Geometry: final body of the model. Coordinates: model frame, mm. Face numbers are marked on the shaded views. A direction names the side the tool comes from. Give positions to 0.01 mm unless a question says otherwise; leave off trailing zeros. Loops run counter-clockwise (first coordinate to the right, second up) from the corner with the lowest first, then second, coordinate; pieces in that order, holes last. Notation, with made-up numbers: (11, 89) -> (21, 89) arc R23 ccw to (21, 116) -> close; hole circle Ø5 at (19.25, 2.25). An arc over 180 degrees is marked (long way). Answer in a Markdown table with one row per item. Add a question column.
1) Line query: line 1 (Z direction, x = 0, y = 24.6); line 2 (Z direction, x = -2.5, y = 0.5); line 3 (X direction, y = -22.5, z = -2.5). Output: solid intervals per line, ascending. Write a range as from..to.
2) Section query B-B (y = -22.5). Return the cut outline in (x, z), plus the area to 3 significant figures.
3) First-contact query: P1, Ø10, axis at y = -2, z = -31.5, coming from the +X side; P2, Ø4, axis at y = 18.5, z = 0.5, coming from the -X side; P3, Ø2.5, axis at y = -20, z = -6, coming from the -X side; P4, Ø12, axis at y = -19.5, z = -26, coming from the -X side. Flat tips, straight axial feed; report the tip coordinate or a pass-through.
4) Section query A-A (x = 0). Give the number of separate pieces and of enclosed holes in the cut face, plus the area to 3 significant figures.
5) Section query D-D (z = -6). Return the cut outline in (x, y), plus the area to 3 significant figures.
6) Section query C-C (x = 14). Return the cut outline in (y, z), plus the area to 3 significant figures.
7) Access query for the marked faces 1, 2, 3 and 4. Directions: +Z, -Z, +X, -X, +Y, -Y. A direction counts if a zero-diameter tool reaches every point of the face in a straight line with its end or side. Return the directions, or none.
8) Draft query along Z for the marked faces 5, 6 and 7. Return one class per face: +Z half, -Z half, draft (parallel to the pull), parting line (faces both ways), or undercut.
```python
from build123d import *

# Parameters (mm, degrees)
SKETCH_1_R           = 20
EXTRUDE_1_DEPTH      = 5
SKETCH_3_W           = 18
SKETCH_3_H           = 8
EXTRUDE_2_DEPTH      = 15
EXTRUDE_3_DEPTH      = 35.22
EXTRUDE_3_DEPTH_BACK = 4.78
SKETCH_4_R           = 20
EXTRUDE_4_DEPTH      = 6
EXTRUDE_4_DEPTH_BACK = 36.43845651
SKETCH_6_R           = 15
SKETCH_10_R          = 8
CUT_EXTRUDE_1_DEPTH  = 6
EXTRUDE_START        = 6
SKETCH_14_R          = 15
EXTRUDE_6_DEPTH      = 6
CUT_EXTRUDE_START    = 6
SKETCH_11_R          = 8
CUT_EXTRUDE_4_DEPTH  = 6
SKETCH_16_R          = 4
CUT_EXTRUDE_5_DEPTH  = 50
SKETCH_23_R          = 4.01
SKETCH_23_R_2        = 3.99
EXTRUDE_7_DEPTH      = 3.22


with BuildPart() as part:
    # Sketch 1 → Extrude 1 (new body)
    with BuildSketch(Plane.XY):
        Circle(SKETCH_1_R)
    extrude(amount=EXTRUDE_1_DEPTH)

    # Sketch 3 → Extrude 2 (add)
    with BuildSketch(Plane.XY.offset(5)):
        with Locations((0, -19.652481849)):
            Rectangle(SKETCH_3_W, SKETCH_3_H)
        with Locations((0, 18.785974665)):
            Rectangle(SKETCH_3_W, SKETCH_3_H)
    extrude(amount=-EXTRUDE_2_DEPTH)

    # Sketch 4 → Extrude 3 (add, two sides: drawn at the far end of the back side and taken through both)
    with BuildSketch(Plane.XZ.offset(-14.785974665).offset(-EXTRUDE_3_DEPTH_BACK)):
        with Locations(Location((0, -22.547246605, 0), (0, 0, 63.25631605))):
            Circle(SKETCH_4_R)
    extrude(amount=EXTRUDE_3_DEPTH + EXTRUDE_3_DEPTH_BACK)

    # Sketch 6 → Extrude 4 (add, two sides: drawn at the far end of the back side and taken through both)
    with BuildSketch(Plane(origin=(0, 19.565974665, 0), x_dir=(1, 0, 0), z_dir=(0, 1, 0)).offset(-EXTRUDE_4_DEPTH_BACK)):
        with Locations(Location((0, 22.272123062, 0), (0, 0, 180))):
            Circle(SKETCH_6_R)
    extrude(amount=EXTRUDE_4_DEPTH + EXTRUDE_4_DEPTH_BACK)

    # Sketch 10 → Cut-Extrude 1 (cut)
    with BuildSketch(Plane(origin=(0, 22.785974665, 0), x_dir=(1, 0, 0), z_dir=(0, 1, 0))):
        with Locations(Location((0, 22.272123062, 0), (0, 0, 180))):
            Circle(SKETCH_10_R)
    extrude(amount=CUT_EXTRUDE_1_DEPTH, mode=Mode.SUBTRACT)

    # Sketch 14 → Extrude 6 (add)
    with BuildSketch(Plane(origin=(0, -20.434025335, 0), x_dir=(-1, 0, 0), z_dir=(0, -1, 0)).offset(EXTRUDE_START)):
        with Locations((0, 22.272123062)):
            Circle(SKETCH_14_R)
    extrude(amount=-EXTRUDE_6_DEPTH)

    # Sketch 11 → Cut-Extrude 4 (cut)
    with BuildSketch(Plane.XZ.offset(23.652481849).offset(CUT_EXTRUDE_START)):
        with Locations(Location((0, -22.272123062, 0), (0, 0, 180))):
            Circle(SKETCH_11_R)
    extrude(amount=-CUT_EXTRUDE_4_DEPTH, mode=Mode.SUBTRACT)

    # Sketch 16 → Cut-Extrude 5 (cut)
    with BuildSketch(Plane(origin=(0, 22.785974665, 0), x_dir=(1, 0, 0), z_dir=(0, 1, 0))):
        with Locations(Location((0, 22.272123062, 0), (0, 0, 270))):
            Circle(SKETCH_16_R)
    extrude(amount=-CUT_EXTRUDE_5_DEPTH, mode=Mode.SUBTRACT)

    # Sketch 23 → Extrude 7 (add)
    with BuildSketch(Plane(origin=(0, 22.785974665, 0), x_dir=(1, 0, 0), z_dir=(0, 1, 0))):
        with Locations((0, 22.272123062)):
            Circle(SKETCH_23_R)
        with Locations(Location((0, 22.272123062, 0), (0, 0, 270))):
            Circle(SKETCH_23_R_2, mode=Mode.SUBTRACT)
    extrude(amount=-EXTRUDE_7_DEPTH)


solid = part.part
```
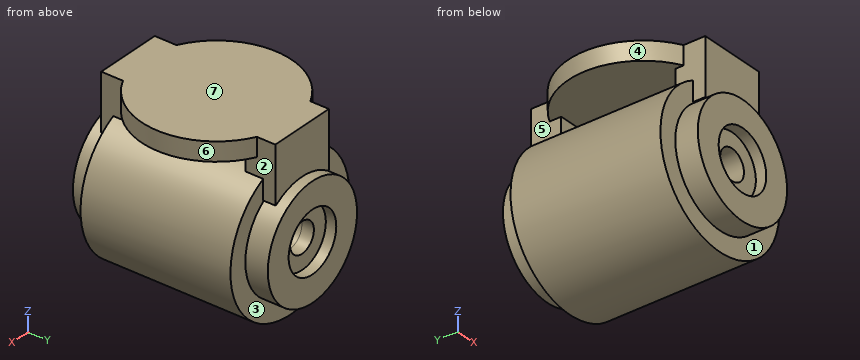
Evaluation:
| question | item | result |
|---|---|---|
| 1 | line 1 | -37.27..-30.27, -14.27..-7.27 |
| 1 | line 2 | -42.39..-25.39, -19.15..-2.7, 0..5 |
| 1 | line 3 | -9..9 |
| 2 | outline | (-9, -10) -> (-8.63, -10) arc R15 ccw (long way) to (8.63, -10) -> (9, -10) -> (9, 5) -> (-9, 5) -> close; hole circle Ø8 at (0, -22.27) |
| 2 | area | 895 mm² |
| 3 | P1 | x = 19.61 |
| 3 | P2 | x = -11.3 |
| 3 | P3 | x = -12.88 |
| 3 | P4 | x = -20 |
| 4 | separate pieces | 2 |
| 4 | enclosed holes | 1 |
| 4 | area | 1,800 mm² |
| 5 | outline | (-11.23, -20.43) -> (-9, -20.43) -> (-9, -23.65) -> (9, -23.65) -> (9, -20.43) -> (11.23, -20.43) -> (11.23, 19.57) -> (9, 19.57) -> (9, 22.79) -> (-9, 22.79) -> (-9, 19.57) -> (-11.23, 19.57) -> close |
| 5 | area | 1,010 mm² |
| 6 | outline | (-26.43, -27.66) -> (-20.43, -27.66) -> (-20.43, -36.83) -> (19.57, -36.83) -> (19.57, -27.66) -> (25.57, -27.66) -> (25.57, -16.89) -> (19.57, -16.89) -> (19.57, -8.26) -> (-20.43, -8.26) -> (-20.43, -16.89) -> (-26.43, -16.89) -> close; (-14.28, 0) -> (14.28, 0) -> (14.28, 5) -> (-14.28, 5) -> close |
| 6 | area | 1,410 mm² |
| 7 | face 1 | -Y |
| 7 | face 2 | +X, +Y |
| 7 | face 3 | +Y |
| 7 | face 4 | +Z, -X |
| 8 | face 5 | undercut |
| 8 | face 6 | draft |
| 8 | face 7 | +Z half |
